Verification items for the finished model (mm, model axes). Give positions to 0.01 mm unless a question says otherwise; leave off trailing zeros. Order: outer loops, then holes, each group sorted by start corner. A loop starts at its lowest first (then second) coordinate and runs counter-clockwise, first axis right, second up.
Autodesk Inventor part; units mm, degrees
ref_plane "YZ Plane" through (0, 0, 0) normal (1, 0, 0) x (0, 1, 0)
ref_plane "XZ Plane" through (0, 0, 0) normal (0, 1, 0) x (-1, 0, 0)
ref_plane "XY Plane" through (0, 0, 0) normal (0, 0, 1) x (1, 0, 0)
sketch "Skizze1" plane through (0, 0, 0) normal (0, 0, 1) x (1, 0, 0)
  line L0 (0, 161) -> (0, -161)
  line L1 (-126, 0) -> (126, 0)
  line L2 (-90, 115) -> (90, 115)
  line L3 (90, 115) -> (90, -115)
  line L4 (90, -115) -> (-90, -115)
  line L5 (-90, -115) -> (-90, 115)
  point P0 (0, 0)
  point P1 (0, 115)
  point P2 (-90, 0)
  dimension "d0" = 230
  dimension "d1" = 180
extrude "Extrusion1" add sketch "Skizze1" along normal blind 4
sketch "Skizze2" plane through (0, 0, 4) normal (0, 0, 1) x (1, 0, 0)
  line L0 (-90, -115) -> (-90, 115)
  line L1 (90, -115) -> (-90, -115)
  line L2 (90, 115) -> (90, -115)
  point P0 (0, 0)
  point P1 (-70, -100)
  point P2 (70, -100)
  dimension "d4" = 20
  dimension "d5" = 20
  dimension "d6" = 15
  dimension "d7" = 15
hole "Bohrung1" at (-70, -100, 4) at (70, -100, 4) direction (0, 0, -1) diameter 6.4 end through all
sketch "Skizze3" plane through (0, 0, 4) normal (0, 0, 1) x (1, 0, 0)
  line L0 (90, -115) -> (-90, -115)
  line L1 (90, 115) -> (90, -115)
  line L2 (90, 115) -> (86, 115)
  line L3 (86, 115) -> (86, -115)
  line L4 (86, -115) -> (90, -115)
  line L5 (90, -115) -> (90, 115)
  point P0 (0, 0)
  dimension "d15" = 4
extrude "Extrusion2" cut sketch "Skizze3" against normal blind 2
sketch "Skizze4" plane through (0, 0, 4) normal (0, 0, 1) x (1, 0, 0)
  line L0 (-90, 115) -> (86, 115)
  line L1 (-90, -115) -> (-90, 115)
  line L2 (-50, 75) -> (50, 75)
  line L3 (50, 75) -> (50, -45)
  line L4 (50, -45) -> (-50, -45)
  line L5 (-50, -45) -> (-50, 75)
  point P0 (0, 0)
  dimension "d18" = 100
  dimension "d19" = 120
  dimension "d20" = 40
  dimension "d21" = 40
extrude "Extrusion3" cut sketch "Skizze4" against normal through all
fillet "Rundung1" radius 10 4 edges at (-50, 75, 2) (50, 75, 2) (50, -45, 2) (-50, -45, 2)
sketch "Skizze5" plane through (0, 0, 4) normal (0, 0, 1) x (1, 0, 0)
  line L0 (-90, -115) -> (-90, 115)
  line L1 (86, -115) -> (-90, -115)
  line L2 (-50, -115) -> (50, -115)
  line L3 (50, -115) -> (50, -85)
  line L4 (50, -85) -> (-50, -85)
  line L5 (-50, -85) -> (-50, -115)
  point P0 (0, 0)
  dimension "d25" = 100
  dimension "d26" = 30
  dimension "d27" = 40
extrude "Extrusion4" cut sketch "Skizze5" against normal through all
fillet "Rundung2" radius 10 2 edges at (-50, -85, 2) (50, -85, 2)
sketch "Skizze6" plane through (0, 0, 0) normal (0, 0, -1) x (-1, 0, 0)
  line L0 (90, -115) -> (50, -115)
  line L1 (90, 115) -> (90, -115)
  line L2 (-90, 115) -> (90, 115)
  line L3 (-90, -115) -> (-90, 115)
  line L4 (-40, -85) -> (40, -85)
  point P0 (0, 0)
  point P1 (-65, 111)
  point P2 (30, 111)
  point P3 (86, 65)
  point P4 (86, -35)
  point P5 (30, -81)
  point P6 (-65, -81)
  dimension "d31" = 60
  dimension "d32" = 4
  dimension "d33" = 25
  dimension "d34" = 50
  dimension "d35" = 4
  dimension "d36" = 4
  dimension "d37" = 80
  dimension "d38" = 4
  dimension "d39" = 60
  dimension "d40" = 4
  dimension "d41" = 25
  dimension "d42" = 4
hole "Bohrung2" at (65, 111, 0) at (-30, 111, 0) at (-86, 65, 0) at (-86, -35, 0) at (-30, -81, 0) at (65, -81, 0) direction (0, 0, 1) diameter 3.2 end through all countersink diameter 6.2 countersink angle 90
sketch "Skizze7" plane through (0, 0, 4) normal (0, 0, 1) x (1, 0, 0)
  line L0 (-49.5, 75) -> (-49.5, 85)
  line L1 (49.5, 85) -> (-49.5, 85)
  line L2 (49.5, 85) -> (49.5, 75)
  line L3 (49.5, 75) -> (-49.5, 75)
  circle A0 centre (-34.5, 80) radius 1.2295
  circle A1 centre (34.5, 80) radius 1.2295
  circle A2 centre (34.5, -50) radius 1.2295
  circle A3 centre (-34.5, -50) radius 1.2295
  line L4 (-49.5, -45) -> (-49.5, -55)
  line L5 (49.5, -55) -> (-49.5, -55)
  line L6 (49.5, -55) -> (49.5, -45)
  line L7 (49.5, -45) -> (-49.5, -45)
  point P0 (0, 0)
hole "Bohrung3" at (-34.5, -50, 4) at (34.5, -50, 4) at (34.5, 80, 4) at (-34.5, 80, 4) direction (0, 0, -1) diameter 3.2 end through all countersink diameter 6.2 countersink angle 90
properties part number "Boden" material "Polycarbonate, Smoke"
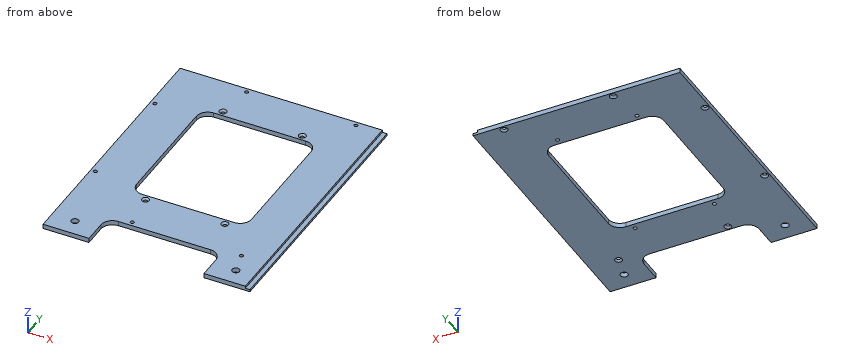
(1) Section check D-D, the plane x = 12.5. Enter the section's corners in (y, z), then the cut area to 3 significant figures.
Solved:
outline: (-85, 0) - (-45, 0) - (-45, 4) - (-85, 4) - close; (75, 0) - (115, 0) - (115, 4) - (75, 4) - close
area: 320 mm2
(2) Go/stop test with flat-tipped pins: pin 1 (2.5 mm diameter, centred on x = 65, y = 111, fed in from -Z); pin 2 (1.5 mm diameter, centred on x = 37.5, z = 3.5, fed in from -Y); pin 3 (1.6 mm diameter, centred on y = -15, z = 3.5, fed in from +X). Record where each tip stops, or that it passes through.
Solved:
pin 1: passes through
pin 2: stops at y = -85
pin 3: stops at x = 86
(3) Scan lines: line 1 (X direction, y = 80, z = 0.7); line 2 (X direction, y = -81, z = 3); line 3 (X direction, y = -100, z = 2.2). Record each from-to range of solid material in increasing order.
Solved:
line 1: x = -90 to -36.1, -32.9 to 32.9, 36.1 to 90
line 2: x = -90 to -31.6, -28.4 to 63.4, 66.6 to 86
line 3: x = -90 to -73.2, -66.8 to -50, 50 to 66.8, 73.2 to 86
(4) Section check C-C, the plane y = 12.5. Enter the section's corners in (x, z).
Solved:
outline: (-90, 0) - (-50, 0) - (-50, 4) - (-90, 4) - close; (50, 0) - (90, 0) - (90, 2) - (86, 2) - (86, 4) - (50, 4) - close
(5) Section check A-A, the plane y = -100. Enter the section's corners in (x, z), then the cut area to 3 significant figures.
Solved:
outline: (-90, 0) - (-73.2, 0) - (-73.2, 4) - (-90, 4) - close; (-66.8, 0) - (-50, 0) - (-50, 4) - (-66.8, 4) - close; (50, 0) - (66.8, 0) - (66.8, 4) - (50, 4) - close; (73.2, 0) - (90, 0) - (90, 2) - (86, 2) - (86, 4) - (73.2, 4) - close
area: 261 mm2
(6) Section check B-B, the plane x = -70. Enter the section's corners in (y, z).
Solved:
outline: (-115, 0) - (-103.2, 0) - (-103.2, 4) - (-115, 4) - close; (-96.8, 0) - (115, 0) - (115, 4) - (-96.8, 4) - close
